Verification items for the finished model (mm, model axes). A direction names the side the tool comes from. Round coordinates to 2 decimals unless told otherwise and drop trailing zeros. Order: outer loops, then holes, each group sorted by start corner. A loop starts at its lowest first (then second) coordinate and runs counter-clockwise, first axis right, second up. Notation, with made-up numbers: (-35, 6) -> (-12, 6) arc R32 cw to (-12, 43) -> close; hole circle Ø4 at (16.25, -18.5). An arc over 180 degrees is marked (long way). Put each result on its own line as item: value.
Autodesk Inventor part; units mm, degrees
ref_plane "YZ Plane" through (0, 0, 0) normal (1, 0, 0) x (0, 1, 0)
ref_plane "XZ Plane" through (0, 0, 0) normal (0, 1, 0) x (-1, 0, 0)
ref_plane "XY Plane" through (0, 0, 0) normal (0, 0, 1) x (1, 0, 0)
sketch "스케치1" plane through (0, 0, 0) normal (0, 1, 0) x (-1, 0, 0)
  line L0 (0, 0) -> (-52, 0)
  line L1 (-52, 0) -> (-52, -52)
  line L2 (-52, -52) -> (0, -52)
  line L3 (0, -52) -> (0, 0)
  line L4 (-52, -5) -> (0, -5)
  line L5 (0, -47) -> (-52, -47)
  dimension "d0" = 52
  dimension "d1" = 52
  dimension "d2" = 5
  dimension "d7" = 5
extrude "돌출1" add sketch "스케치1" along normal blind 5 contours L3 L5 L1 L4
extrude "돌출2" add sketch "스케치1" along normal blind 47 contours L3 L4 L1 L0 | L3 L2 L1 L5
sketch "스케치2" plane through (0, 0, 0) normal (0, -1, 0) x (1, 0, 0)
  line L0 (52, -52) -> (0, -52)
  line L1 (52, -52) -> (52, -32)
  line L2 (52, 0) -> (52, -52)
  line L3 (52, -52) -> (42, -52)
  line L4 (42, -52) -> (52, -32)
  line L5 (42, -52) -> (32.1613, -71.6774)
  line L6 (32.1613, -71.6774) -> (64.3607, -7.2786)
  line L7 (64.3607, -7.2786) -> (21.4282, 14.1876)
  line L8 (21.4282, 14.1876) -> (-10.7712, -50.2111)
  line L9 (-10.7712, -50.2111) -> (32.1613, -71.6774)
  line L10 (-5.4046, -48.4223) -> (23.217, 8.821)
  line L11 (23.217, 8.821) -> (58.9941, -9.0675)
  line L12 (58.9941, -9.0675) -> (30.3724, -66.3108)
  line L13 (33.9502, -68.0997) -> (-5.4046, -48.4223)
  line L14 (60.783, -5.4898) -> (55.8636, -15.3285)
  line L15 (55.8636, -15.3285) -> (59.4413, -17.1173)
  point P0 (0, 0)
  dimension "d0" = 52
  dimension "d1" = 52
  dimension "d2" = 5
  dimension "d7" = 5
  dimension "d8" = 20
  dimension "d9" = 10
  dimension "d10" = 22
  dimension "d11" = 72
  dimension "d12" = 48
  dimension "d13" = 4
  dimension "d14" = 11
extrude "돌출3" add sketch "스케치2" along normal blind 4 contours L5 L13 L12 L0 | L0 L12 L2 L4 | L2 L12 L15 L6 | L12 L13 L0 | L0 L13 L10 L11 L2 L12 | L2 L11 L12
extrude "돌출4" add sketch "스케치2" along normal blind 27 contours L5 L9 L8 L7 L2 L11 L10 L13 | L2 L7 L14 L11
sketch "스케치3" plane through (58.9941, -27, -9.0675) normal (-0.4472136, 0, -0.8944272) x (-0.8944272, 0, 0.4472136)
  line L0 (0, 23) -> (0, 0)
  line L1 (0, 0) -> (0, 4)
  line L2 (0, 4) -> (40, 4)
  line L3 (40, 23) -> (40, 0)
  line L4 (40, 0) -> (0, 0)
  point P0 (56.821, 27)
  dimension "d19" = 4
extrude "돌출5" add sketch "스케치3" along normal blind 52
sketch "스케치4" plane through (0, -27, 0) normal (0, -1, 0) x (1, 0, 0)
  line L0 (32.1613, -71.6774) -> (33.9502, -68.0997)
  line L1 (33.9502, -68.0997) -> (-5.4046, -48.4223)
  line L2 (-5.4046, -48.4223) -> (-0.0381, -37.6892)
  line L3 (35.739, -55.5777) -> (-0.0381, -37.6892)
  line L4 (60.783, -5.4898) -> (35.739, -55.5777)
  line L5 (60.783, -5.4898) -> (21.4282, 14.1876)
  line L6 (21.4282, 14.1876) -> (-10.7712, -50.2111)
  line L7 (-10.7712, -50.2111) -> (32.1613, -71.6774)
  line L8 (-0.0381, -37.6892) -> (-3.6158, -35.9003)
  line L9 (32.1613, -71.6774) -> (42, -52)
  line L10 (33.9502, -68.0997) -> (32.1613, -71.6774)
  line L11 (32.1613, -71.6774) -> (-10.7712, -50.2111)
  line L12 (-3.6158, -35.9003) -> (-0.0381, -37.6892)
  point P0 (0, 0)
extrude "돌출6" cut sketch "스케치4" against normal blind 10 contours L7 L6 L8 L2 L1 L0
sketch "스케치5" plane through (0, 47, 0) normal (0, 0, 1) x (1, 0, 0)
  line L0 (0, -47) -> (14.3344, -47)
  line L1 (14.3344, -47) -> (49.8034, -47)
  line L2 (49.8034, -47) -> (52, -47)
  line L3 (52, -47) -> (52, 0)
  line L4 (0, 0) -> (52, 0)
  line L5 (0, -47) -> (0, 0)
  circle A0 centre (26, -20.574) radius 4.5
  point P0 (26, 0)
  dimension "d24" = 9
  dimension "d25" = 16.074
extrude "돌출7" cut sketch "스케치5" against normal blind 100 contours A0
properties part number "camera_case"
Item 1: Material ranges on L1, parallel to Y at x = 26, z = -2.9; L2, parallel to Z at x = 34, y = 22.5; L3, parallel to Y at x = 47.5, z = -29, recorded low to high. Write a range as [from, to].
Check sheet entries:
L1: y = [-27, -23], [-4, 21.93], [30.93, 47]
L2: z = [-52, -47], [-5, 0]
L3: y = [-27, -23], [-4, 5]
Item 2: Gauge pin test, flat ends, axial feed: pin 1 Ø12.5 at (x, y) = (32.5, 26) entering from -Z; pin 2 Ø2 at (x, y) = (32.5, -4.5) entering from +Z; pin 3 Ø5 at (x, y) = (32.5, 31.5) entering from +Z; pin 4 Ø1.5 at (x, y) = (25, 29.5) entering from +Z. Record the tip position at first contact, or that the pin passes through.
Check sheet entries:
pin 1: stops at z = -52
pin 2: stops at z = 9.15
pin 3: stops at z = 0
pin 4: passes through
Item 3: Section check C-C on x = 26. Record the boundary of the cut face in (y, z), then the cut area to 3 significant figures.
Check sheet entries:
outline: (-27, -50.71) -> (-23, -50.71) -> (-23, 7.43) -> (-4, 7.43) -> (-4, -64.12) -> (-17, -64.12) -> (-17, -68.6) -> (0, -68.6) -> (0, -52) -> (21.93, -52) -> (21.93, -47) -> (5, -47) -> (5, -5) -> (21.93, -5) -> (21.93, 0) -> (0, 0) -> (0, 11.9) -> (-27, 11.9) -> close; (30.93, -52) -> (47, -52) -> (47, -47) -> (30.93, -47) -> close; (30.93, -5) -> (47, -5) -> (47, 0) -> (30.93, 0) -> close
area: 1,310 mm^2
Item 4: Section check D-D on x = 44.5. Record the boundary of the cut face in (y, z), then the cut area to 3 significant figures.
Check sheet entries:
outline: (-27, -38.06) -> (-23, -38.06) -> (-23, -1.82) -> (-4, -1.82) -> (-4, -47) -> (0, -47) -> (0, -52) -> (47, -52) -> (47, -47) -> (5, -47) -> (5, -5) -> (47, -5) -> (47, 0) -> (0, 0) -> (0, 2.65) -> (-27, 2.65) -> close
area: 1,130 mm^2
Item 5: Release check for a two-part mould opening along Z. For faces 6 (the flat face through (8.706, -13.367, -20.201)), 7 (the flat face through (0, 4, -28)), 8 (the flat face through (44, -3, -48)) record: +Z half, -Z half, draft (parallel to the pull), parting line (faces both ways), or undercut.
Check sheet entries:
face 6: undercut
face 7: draft
face 8: -Z half
Item 6: Section check B-B on z = -41. Record the boundary of the cut face in (x, y), then the cut area to 3 significant figures.
Check sheet entries:
outline: (-6.17, -17) -> (-1.69, -17) -> (-1.69, -4) -> (47.5, -4) -> (47.5, 0) -> (52, 0) -> (52, 5) -> (0, 5) -> (0, 0) -> (-6.17, 0) -> close; (6.58, -27) -> (43.03, -27) -> (43.03, -23) -> (6.58, -23) -> close
area: 679 mm^2
Item 7: Section check A-A on y = 8. Record the boundary of the cut face in (x, z), then the cut area to 3 significant figures.
Check sheet entries:
outline: (0, -52) -> (52, -52) -> (52, -47) -> (0, -47) -> close; (0, -5) -> (52, -5) -> (52, 0) -> (0, 0) -> close
area: 520 mm^2
Item 8: Tool access check on faces 1 (the flat face through (26, 18, 0)), 2 (the flat face through (30, -23, -23)), 3 (the flat face through (14.55, -10.41, -58.4)), 4 (the flat face through (40.86, -13.37, 0)), 5 (the flat face through (26, 21, -5)). Record the directions out of +Z, -Z, +X, -X, +Y, -Y that give a thin tool (end or side, any length) a straight path to the whole face; none if there is none.
Check sheet entries:
face 1: +Z, +X, -X, +Y
face 2: -Z
face 3: +X, -Y
face 4: none
face 5: +X, -X, +Y
